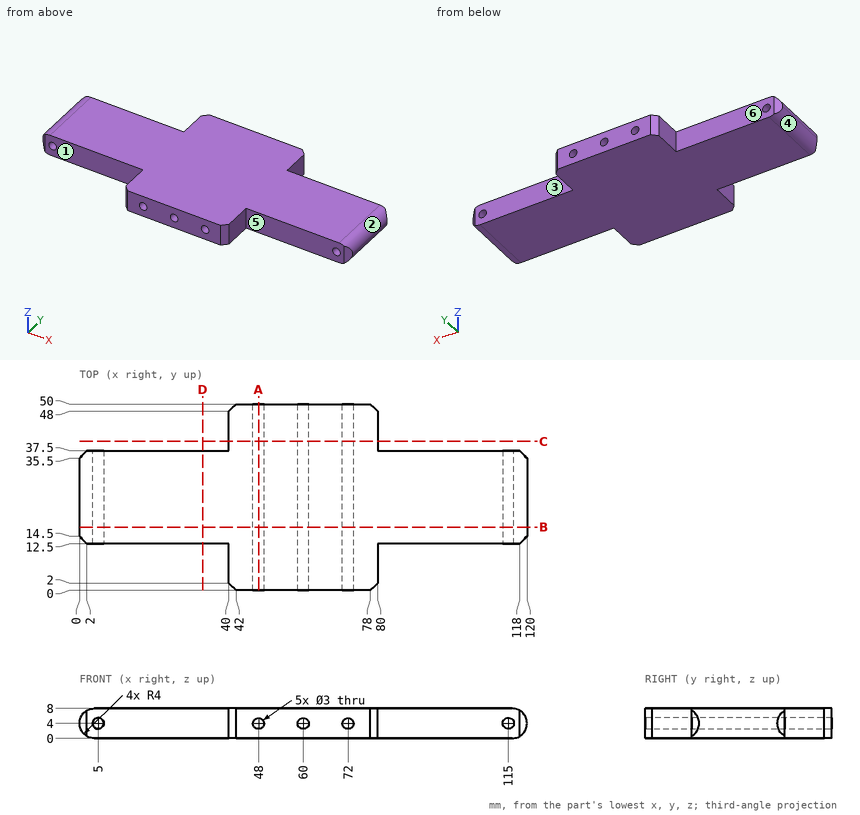
The drawing under review shows one solid part. Ordinate dimensions are in mm from its lowest x, y, z. A direction names the side the tool comes from. Round coordinates to 2 decimals unless told otherwise and drop trailing zeros. Loops run counter-clockwise (first coordinate to the right, second up) from the corner with the lowest first, then second, coordinate; pieces in that order, holes last. Notation, with made-up numbers: (65.25, 1) -> (120.25, 1) arc R7 cw to (120.25, 8) -> close; hole circle Ø2 at (64, 73.5). An arc over 180 degrees is marked (long way). Answer in a Markdown table with one row per item.
1) Wall thickness on line 1 along X through (y, z) = (11, 4); line 2 along X through (y, z) = (11, 2.75); line 3 along Z through (x, y) = (5, 19): over which ranges is each line inside the solid? List them lowest first.
Taken from the geometry:
| item | result |
|---|---|
| line 1 | x = 40 to 46.5, 49.5 to 58.5, 61.5 to 70.5, 73.5 to 80 |
| line 2 | x = 40 to 47.17, 48.83 to 59.17, 60.83 to 71.17, 72.83 to 80 |
| line 3 | z = 0 to 2.5, 5.5 to 8 |
2) Consider section A-A, the plane x = 48. Write out the cut boundary in (y, z), plus the area to 3 significant figures.
Taken from the geometry:
| item | result |
|---|---|
| outline | (0, 0) -> (50, 0) -> (50, 2.5) -> (0, 2.5) -> close; (0, 5.5) -> (50, 5.5) -> (50, 8) -> (0, 8) -> close |
| area | 250 mm² |
3) Draft analysis for pull direction Y (two halves, no side actions). For the marked faces 4, 5 and 6, state which applies: pulls with the +Y half, pulls with the -Y half, needs draft (parallel to the pull), parting line crosses it, or undercut.
Taken from the geometry:
| item | result |
|---|---|
| face 4 | needs draft |
| face 5 | pulls with the -Y half |
| face 6 | pulls with the +Y half |
4) Consider section D-D, the plane x = 33. Write out the cut boundary in (y, z), plus the area to 3 significant figures.
Taken from the geometry:
| item | result |
|---|---|
| outline | (12.5, 0) -> (37.5, 0) -> (37.5, 8) -> (12.5, 8) -> close |
| area | 200 mm² |
5) For pin 1 Ø4 at (x, z) = (5, 4) entering from +Y; pin 2 Ø4 at (y, z) = (9.5, 3) entering from +X; pin 3 Ø2.5 at (x, z) = (100, 5) entering from -Y; pin 4 Ø2.5 at (x, z) = (48, 4) entering from -Y, all flat-tipped, find the tip position at first contact; note any pin that passes through.
Taken from the geometry:
| item | result |
|---|---|
| pin 1 | stops at y = 37.5 |
| pin 2 | stops at x = 80 |
| pin 3 | stops at y = 12.5 |
| pin 4 | passes through |
6) Tool access review of the marked faces 1, 2 and 3: name each direction out of +Z, -Z, +X, -X, +Y, -Y from which nothing blocks a thin tool from reaching the whole face with its end or side.
Taken from the geometry:
| item | result |
|---|---|
| face 1 | +Z, -Z, -X, -Y |
| face 2 | +Z, +X, +Y, -Y |
| face 3 | +Z, -Z, +X, +Y |
7) Consider section B-B, the plane y = 17. Count the separate pieces of the cut face and the enclosed holes in it, plus the area to 3 significant figures.
Taken from the geometry:
| item | result |
|---|---|
| separate pieces | 1 |
| enclosed holes | 5 |
| area | 911 mm² |
8) Consider section C-C, the plane y = 40. Write out the cut boundary in (x, z), plus the area to 3 significant figures.
Taken from the geometry:
| item | result |
|---|---|
| outline | (40, 0) -> (80, 0) -> (80, 8) -> (40, 8) -> close; hole circle Ø3 at (48, 4); hole circle Ø3 at (60, 4); hole circle Ø3 at (72, 4) |
| area | 299 mm² |
